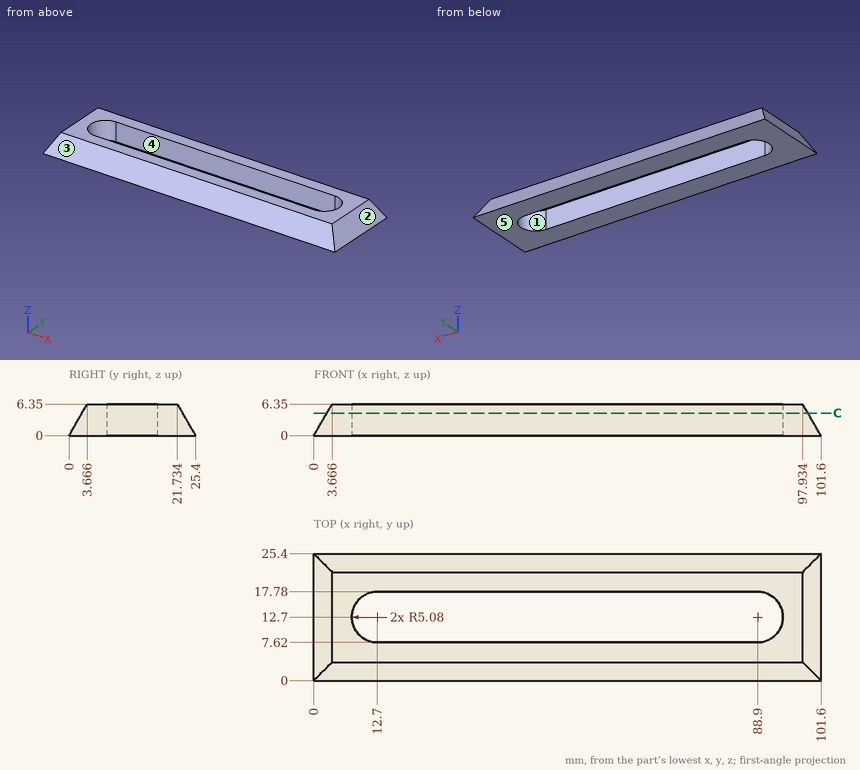
The figure shows three views and two pictorial views of one solid part (mm, origin at its lowest corner). Answer the questions. A direction names the side the tool comes from. Give positions to 0.01 mm unless a question says otherwise; leave off trailing zeros. Order: outer loops, then holes, each group sorted by start corner. A loop starts at its lowest first (then second) coordinate and runs counter-clockwise, first axis right, second up. Notation, with made-up numbers: M -9.5,41 L 38.5,41 A20 cw 38.5,72 Z; hole C 53,38.25 d4. An arc over 180 degrees is marked long. Return JSON: item names as keys, results as strings.
Q1. The mould has two halves that part along X. Classify the marked faces 1, 2 and 3: pulls with the +X half, pulls with the -X half, needs draft (parallel to the pull), parting line crosses it, or undercut.
Answer below:
{"face 1": "undercut", "face 2": "pulls with the +X half", "face 3": "needs draft"}
Q2. Find section C-C, the plane z = 4.5. Write down the section's boundary in (x, y).
Answer below:
{"outline": "M 2.6,2.6 L 99,2.6 L 99,22.8 L 2.6,22.8 Z; hole M 12.7,7.62 L 88.9,7.62 A5.08 ccw 88.9,17.78 L 12.7,17.78 A5.08 ccw Z"}
Q3. Which of the six approach directions +Z, -Z, +X, -X, +Y, -Y give full straight-line access (tool end or side, diameter ignored) to the marked faces 4 and 5?
Answer below:
{"face 4": "+Z, -Z", "face 5": "-Z, +X, -X, +Y, -Y"}
Q4. Find the intervals of material crossed by line 1 along Y through (x, z) = (27, 5.25); line 2 along Y through (x, z) = (38, 5.5) (1 decimal); line 3 along X through (y, z) = (10.5, 2.25), in increasing order. Write a range as [from, to].
Answer below:
{"line 1": "y = [3.03, 7.62], [17.78, 22.37]", "line 2": "y = [3.2, 7.6], [17.8, 22.2]", "line 3": "x = [1.3, 8.12], [93.48, 100.3]"}
Q5. Each of these flat-tipped pins is pushed along its axis until it touches: pin 1 (2 mm diameter, centred on x = 28, z = 2, fed in from -Y); pin 2 (3 mm diameter, centred on x = 60.5, z = 2, fed in from -Y). Where does it stop, or does it pass through?
Answer below:
{"pin 1": "stops at y = 0.58", "pin 2": "stops at y = 0.29"}
